Design review of the part shown in the three views and the two pictorial views. Dimensions are in mm from the part's minimum x, y and z. Round coordinates to 2 decimals unless told otherwise and drop trailing zeros. Loops run counter-clockwise (first coordinate to the right, second up) from the corner with the lowest first, then second, coordinate; pieces in that order, holes last. Notation, with made-up numbers: (26, 21.5) -> (38, 21.5) arc R18 cw to (38, 36.5) -> close; hole circle Ø10 at (35.5, 49.5). An arc over 180 degrees is marked (long way). Use a Markdown table: item, result. Add a question column.
1) Consider section D-D on z = 0.3. Give the boundary of the cut face in (x, y).
2) Consider section A-A on x = 44. Give the boundary of the cut face in (y, z).
3) Insertion check: pin 1 (2 mm diameter, centred on x = 44, y = 33.5, fed in from +Z); pin 2 (0.8 mm diameter, centred on y = 31.5, z = 0.5, fed in from +X). Each pin has a flat end and moves straight along its axis. Give the tip position at first contact, or say it passes through.
4) Wall thickness on probe 1 along Y at (x, z) = (44, 0.95); probe 2 along Y at (x, z) = (10, 0.6); probe 3 along Y at (x, z) = (28, 0.15): over which ranges is each line inside the solid? List them lowest first.
5) Consider section B-B on y = 27.5. Give the boundary of the cut face in (x, z), plus the area to 3 significant figures.
6) Consider section C-C on x = 27.5. Give the boundary of the cut face in (y, z), plus the area to 3 significant figures.
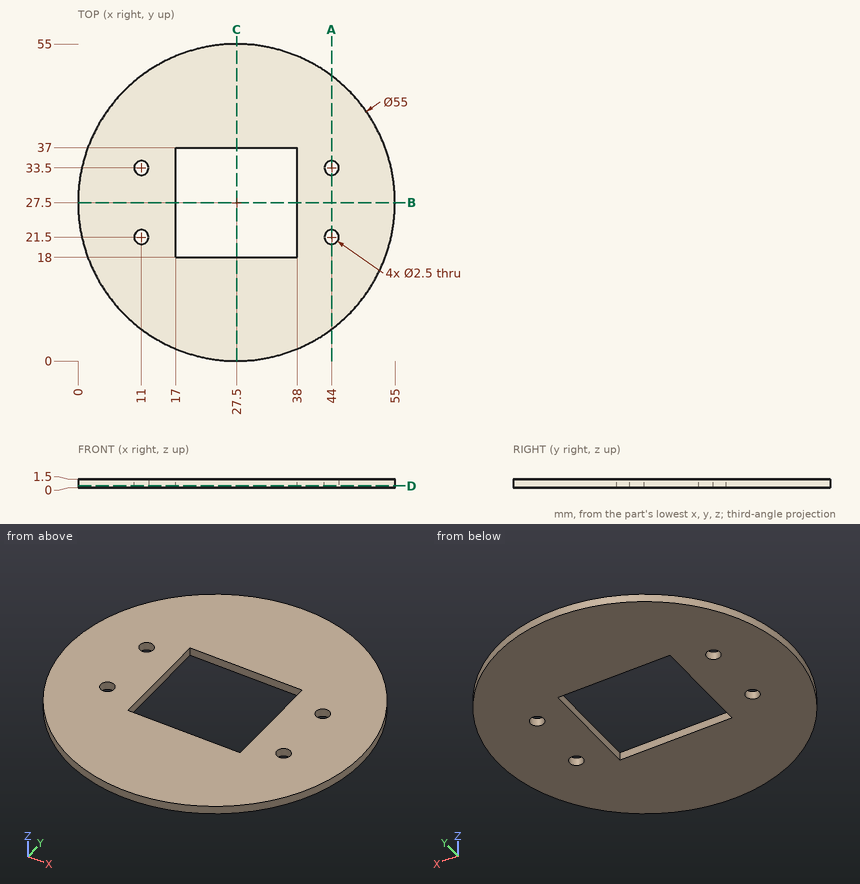
Result set:
| question | item | result |
|---|---|---|
| 1 | outline | circle Ø55 at (27.5, 27.5); hole circle Ø2.5 at (11, 21.5); hole circle Ø2.5 at (11, 33.5); hole (17, 18) -> (38, 18) -> (38, 37) -> (17, 37) -> close; hole circle Ø2.5 at (44, 21.5); hole circle Ø2.5 at (44, 33.5) |
| 2 | outline | (5.5, 0) -> (20.25, 0) -> (20.25, 1.5) -> (5.5, 1.5) -> close; (22.75, 0) -> (32.25, 0) -> (32.25, 1.5) -> (22.75, 1.5) -> close; (34.75, 0) -> (49.5, 0) -> (49.5, 1.5) -> (34.75, 1.5) -> close |
| 3 | pin 1 | through |
| 3 | pin 2 | x = 54.76 |
| 4 | probe 1 | 5.5 to 20.25, 22.75 to 32.25, 34.75 to 49.5 |
| 4 | probe 2 | 6.29 to 20.75, 22.25 to 32.75, 34.25 to 48.71 |
| 4 | probe 3 | 0 to 18, 37 to 55 |
| 5 | outline | (0, 0) -> (17, 0) -> (17, 1.5) -> (0, 1.5) -> close; (38, 0) -> (55, 0) -> (55, 1.5) -> (38, 1.5) -> close |
| 5 | area | 51.0 mm2 |
| 6 | outline | (0, 0) -> (18, 0) -> (18, 1.5) -> (0, 1.5) -> close; (37, 0) -> (55, 0) -> (55, 1.5) -> (37, 1.5) -> close |
| 6 | area | 54.0 mm2 |
